For this review, take the finished solid that the model builds, in its own axes (mm). Face numbers are marked on the shaded views. A direction names the side the tool comes from. Give positions to 0.01 mm unless a question says otherwise; leave off trailing zeros. Order: outer loops, then holes, each group sorted by start corner. A loop starts at its lowest first (then second) coordinate and runs counter-clockwise, first axis right, second up. Notation, with made-up numbers: (50, 68.25) -> (73, 68.25) arc R18 cw to (73, 76.25) -> close; hole circle Ø7 at (-35, 79). An arc over 180 degrees is marked (long way). One line per item, written item: value. Start each with the question number.
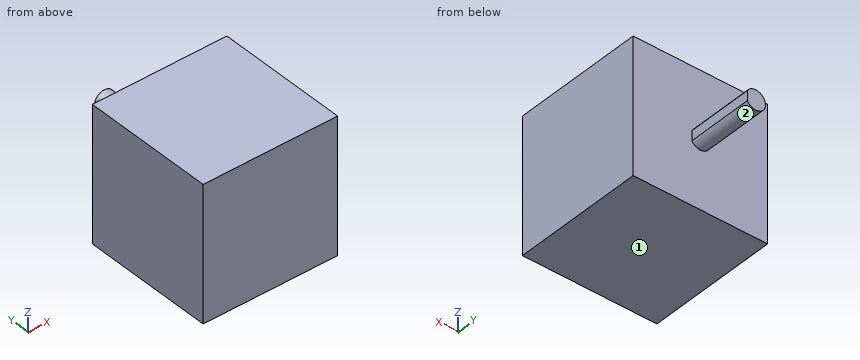
from build123d import *

# Parameters (mm, degrees)
SKETCH1_W           = 55
SKETCH1_H           = 55
BOSS_EXTRUDE1_DEPTH = 54
SKETCH2_R           = 4
BOSS_EXTRUDE2_DEPTH = 27
CUT_EXTRUDE1_DEPTH  = 27


with BuildPart() as part:
    # Sketch1 → Boss-Extrude1 (new body)
    with BuildSketch(Plane(origin=(0, 0, 0), x_dir=(1, 0, 0), z_dir=(0, 1, 0))):
        Rectangle(SKETCH1_W, SKETCH1_H)
    extrude(amount=BOSS_EXTRUDE1_DEPTH)

    # Sketch2 → Boss-Extrude2 (add)
    with BuildSketch(Plane(origin=(0, 54, 0), x_dir=(1, 0, 0), z_dir=(0, 1, 0))):
        with Locations(Location((0, 0, 0), (0, 0, 90))):
            Circle(SKETCH2_R)
    extrude(amount=BOSS_EXTRUDE2_DEPTH)

    # Sketch3 → Cut-Extrude1 (cut)
    with BuildSketch(Plane(origin=(0, 81, 0), x_dir=(1, 0, 0), z_dir=(0, 1, 0))):
        Polygon((3.464101615, 2), (3.464101615, -2), (4.924902358, -3.067380236), (7.380842693, 1.390151472), align=None)
    extrude(amount=-CUT_EXTRUDE1_DEPTH, mode=Mode.SUBTRACT)


solid = part.part
Q1. For pin 1 Ø4.5 at (y, z) = (72, 0) entering from +X; pin 2 Ø1 at (x, z) = (-20.5, -8.5) entering from +Y; pin 3 Ø4 at (x, y) = (5.5, 56.5) entering from +Z, all flat-tipped, find the tip position at first contact; note any pin that passes through.
Q2. For line 1 along Y through (x, z) = (6.5, 12); line 2 along Z through (x, y) = (2.5, 61), list the stretches that pass through material, from the lowest coordinate up.
Q3. Take a section at D-D (z = -20.5). State the section outline as (x, y) points, and give its area (3 significant figures).
Q4. Take a section at C-C (y = 60). State the section outline as (x, z) points, and give its area (3 significant figures).
Q5. For the marked faces 1 and 2, list the 3-axis set-ups (+Z, -Z, +X, -X, +Y, -Y) from which the entire face can be reached by the end or side of a thin tool; tool diameter is ignored.
Q6. Take a section at B-B (z = 0). State the section outline as (x, y) points, and give its area (3 significant figures).
Q7. Take a section at A-A (x = 0). State the section outline as (y, z) points.
Answers below:
1. pin 1: stops at x = 3.46
1. pin 2: stops at y = 54
1. pin 3: passes through
2. line 1: y = 0 to 54
2. line 2: z = -3.12 to 3.12
3. outline: (-27.5, 0) -> (27.5, 0) -> (27.5, 54) -> (-27.5, 54) -> close
3. area: 2,970 mm²
4. outline: (3.46, -2) -> (3.46, 2) arc R4 ccw (long way) to start
4. area: 48.8 mm²
5. face 1: -Z, +X, -X, +Y, -Y
5. face 2: +Y
6. outline: (-27.5, 0) -> (27.5, 0) -> (27.5, 54) -> (3.46, 54) -> (3.46, 81) -> (-4, 81) -> (-4, 54) -> (-27.5, 54) -> close
6. area: 3,170 mm²
7. outline: (0, -27.5) -> (54, -27.5) -> (54, -4) -> (81, -4) -> (81, 4) -> (54, 4) -> (54, 27.5) -> (0, 27.5) -> close
